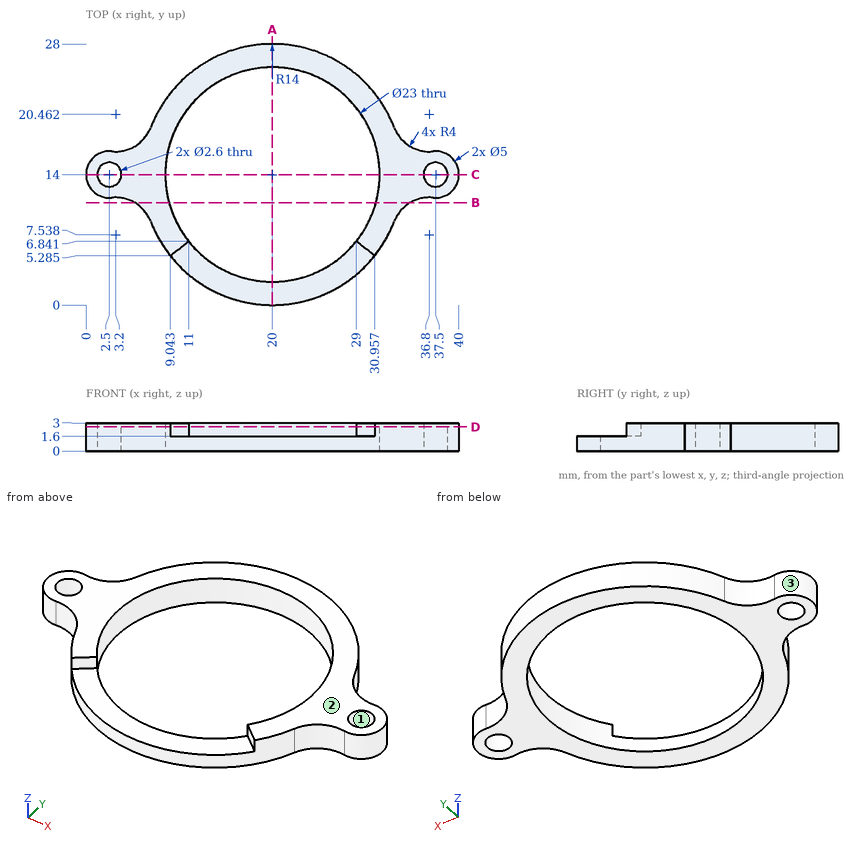
Verification items for this drawing (mm, ordinates from the low corner). Give positions to 0.01 mm unless a question says otherwise; leave off trailing zeros. Write each loop counter-clockwise with the first axis right and the second up, starting at its lowest first coordinate (ties: lowest second). Pieces come first, ordered by that corner, then holes. Notation, with made-up numbers: (-27.5, 30.5) - (10.5, 30.5) arc R17 ccw to (10.5, 36.5) - close; hole circle Ø7 at (46.25, -20.75). An arc over 180 degrees is marked (long way). Answer as CSV lines item,"result". Start each with the question number.
1. Sectioned sample at A-A (x = 20). Record the boundary of the cut face in (y, z).
2. Sectioned sample at D-D (z = 2.6). Record the boundary of the cut face in (x, y) (1 decimal).
3. Sectioned sample at B-B (y = 11). Record the boundary of the cut face in (x, z).
4. Draft check along Y on the marked faces 1, 2 and 3. Enter one of: pulls with the +Y half, pulls with the -Y half, needs draft (parallel to the pull), parting line crosses it, or undercut.
5. Sectioned sample at C-C (y = 14). Record the boundary of the cut face in (x, z).
6. Thickness scan on line 1 (Y direction, x = 2.5, z = 2); line 2 (Y direction, x = 20, z = 0.8); line 3 (X direction, y = 13.25, z = 0.65) (1 decimal). Record the ranges inside material, lowest first.
7. Depth check by flat-ended pin: pin 1 (2 mm diameter, centred on x = 2.5, y = 14, fed in from +Z). Enter the tip coordinate at first touch or a pass-through.
Derived:
1,outline,"(0, 0) - (2.5, 0) - (2.5, 1.6) - (0, 1.6) - close; (25.5, 0) - (28, 0) - (28, 3) - (25.5, 3) - close"
2,outline,"(2.8, 11.5) arc R4 cw to (6.9, 9) arc R14 ccw to (9, 5.3) - (11, 6.8) arc R11.5 cw (long way) to (29, 6.8) - (31, 5.3) arc R14 ccw to (33.1, 9) arc R4 cw to (37.2, 11.5) arc R2.5 ccw (long way) to (37.2, 16.5) arc R4 cw to (33.1, 19) arc R14 ccw to (6.9, 19) arc R4 cw to (2.8, 16.5) arc R2.5 ccw (long way) to start; hole circle Ø2.6 at (2.5, 14); hole circle Ø2.6 at (37.5, 14)"
3,outline,"(5.2, 0) - (8.9, 0) - (8.9, 3) - (5.2, 3) - close; (31.1, 0) - (34.8, 0) - (34.8, 3) - (31.1, 3) - close"
4,face 1,"undercut"
4,face 2,"needs draft"
4,face 3,"parting line crosses it"
5,outline,"(0, 0) - (1.2, 0) - (1.2, 3) - (0, 3) - close; (3.8, 0) - (8.5, 0) - (8.5, 3) - (3.8, 3) - close; (31.5, 0) - (36.2, 0) - (36.2, 3) - (31.5, 3) - close; (38.8, 0) - (40, 0) - (40, 3) - (38.8, 3) - close"
6,line 1,"11.5 to 12.7, 15.3 to 16.5"
6,line 2,"0 to 2.5, 25.5 to 28"
6,line 3,"0.1 to 1.4, 3.6 to 8.5, 31.5 to 36.4, 38.6 to 39.9"
7,pin 1,"through"
